```python
from build123d import *

# Parameters (mm, degrees)
BOSS_EXTRUDE1_DEPTH     = 6.35
F_3_8_CLEARANCE_HOLE1_D = 10.31748
F_1_4_CLEARANCE_HOLE1_D = 7.14248


with BuildPart() as part:
    # Sketch1 → Boss-Extrude1 (new body)
    with BuildSketch(Plane.XY):
        Polygon((-49.2125, 113.079516789), (49.2125, 113.079516789), (122.535984187, -13.920483211), (-122.535984187, -13.920483211), align=None)
    extrude(amount=BOSS_EXTRUDE1_DEPTH)

    # 3/8 Clearance Hole1 (through all)
    with Locations(Plane.XY.offset(6.35)):
        with Locations((0, 78.805444667), (0, 8.955444667)):
            Hole(F_3_8_CLEARANCE_HOLE1_D / 2)

    # 1/4 Clearance Hole1 (through all)
    with Locations(Plane.XY.offset(6.35)):
        with Locations((65.710283942, 1.954516789), (56.838608029, 80.820710219)):
            f_1_4_clearance_hole1 = Hole(F_1_4_CLEARANCE_HOLE1_D / 2)

    # Mirror1: 1/4 Clearance Hole1 across plane
    add(f_1_4_clearance_hole1.mirror(Plane(origin=(0, 0, 0), x_dir=(0, 0, 1), z_dir=(1, 0, 0))), mode=Mode.SUBTRACT)


solid = part.part
```
CAD build for the part. Positions are in the model's coordinates, mm. Round coordinates to 2 decimals unless told otherwise and drop trailing zeros. Order: outer loops, then holes, each group sorted by start corner. A loop starts at its lowest first (then second) coordinate and runs counter-clockwise, first axis right, second up. Notation, with made-up numbers: (85.25, -27.75) - (139.25, -27.75) arc R30 cw to (139.25, 10.25) - close; hole circle Ø6 at (35.5, 31). An arc over 180 degrees is marked (long way). Answer as CSV lines item,"result". Start each with the question number.
1. Saw through at B-B, the plane z = 4.75. Write the cut outline in (x, y), and give its area (3 significant figures).
2. Pull direction Y, two halves, no side cores. Call faces 1 (the face through (-62.41, 0.59, 3.13)), 2 (the face through (-1, 113.08, 3)), 3 (the face through (2, 36, 0)): +Y half, -Y half, draft (parallel to the pull), parting line (faces both ways), or undercut.
3. Saw through at A-A, the plane x = 0. Write the cut outline in (y, z), and give its area (3 significant figures).
4. Drill centre lines: L1, parallel to Y at x = 0, z = 4.5; L2, parallel to X at y = 80.5, z = 3.25; L3, parallel to X at y = 0, z = 3.25. Where is each one in solid material? Low to high. Write a range as [from, to].
5. Saw through at C-C, the plane y = 69. Write the cut outline in (x, z).
6. Saw through at D-D, the plane x = 103. Write the cut outline in (y, z), and give its area (3 significant figures).
Model answer:
1,outline,"(-122.54, -13.92) - (122.54, -13.92) - (49.21, 113.08) - (-49.21, 113.08) - close; hole circle Ø7.14 at (-65.71, 1.95); hole circle Ø7.14 at (-56.84, 80.82); hole circle Ø10.32 at (0, 8.96); hole circle Ø10.32 at (0, 78.81); hole circle Ø7.14 at (56.84, 80.82); hole circle Ø7.14 at (65.71, 1.95)"
1,area,"21,500 mm²"
2,face 1,"undercut"
2,face 2,"+Y half"
2,face 3,"draft"
3,outline,"(-13.92, 0) - (3.8, 0) - (3.8, 6.35) - (-13.92, 6.35) - close; (14.11, 0) - (73.65, 0) - (73.65, 6.35) - (14.11, 6.35) - close; (83.96, 0) - (113.08, 0) - (113.08, 6.35) - (83.96, 6.35) - close"
3,area,"675 mm²"
4,L1,"y = [-13.92, 3.8], [14.11, 73.65], [83.96, 113.08]"
4,L2,"x = [-68.02, -60.4], [-53.28, -4.87], [4.87, 53.28], [60.4, 68.02]"
4,L3,"x = [-114.5, -68.7], [-62.72, 62.72], [68.7, 114.5]"
5,outline,"(-74.66, 0) - (74.66, 0) - (74.66, 6.35) - (-74.66, 6.35) - close"
6,outline,"(-13.92, 0) - (19.92, 0) - (19.92, 6.35) - (-13.92, 6.35) - close"
6,area,"215 mm²"
